Design review of the part built by this model. Coordinates are the model's own, in mm. Coordinates: 2 decimals unless noted, no trailing zeros. Loops run counter-clockwise (first coordinate to the right, second up) from the corner with the lowest first, then second, coordinate; pieces in that order, holes last.
Q1. Add section C-C on x = -8. Give the boundary of the cut face in (y, z) (3 decimals), and give its area (3 significant figures).
Q2. Add section D-D on y = 35.5. Give the boundary of the cut face in (x, z) (3 decimals), and give its area (3 significant figures).
Q3. For P1, Ø13, axis at x = 0, y = 0, coming from the +Z side; P2, Ø4, axis at x = -53.74, y = 48.92, coming from the +Z side; P3, Ø5, axis at x = -40, y = 0, coming from the +Z side; P4, Ø6, axis at x = 0, y = -8, coming from the +Z side (3 decimals), all flat-tipped, find the tip position at first contact; note any pin that passes through.
Q4. Add section B-B on y = 8. Give the boundary of the cut face in (x, z) (3 decimals), and give its area (3 significant figures).
Q5. Wall thickness on probe 1 along X at (y, z) = (47, -0.3); probe 2 along Y at (x, z) = (-68, -1.2); probe 3 along Y at (x, z) = (-57, -1.9): over which ranges is each line inside the solid? List them lowest first.
Q6. Draft analysis for pull direction Y (two halves, no side actions). For faces 1 (the face through (16, 7, -2)), 2 (the face through (-51, 54.5, -2)), 3 (the face through (-67.64, 48.99, -2.37)), state which applies: released by +Y, released by -Y, zero draft, split by the parting line, or undercut.
Q7. Add section A-A on x = -64. Give the boundary of the cut face in (y, z) (3 decimals), and give its area (3 significant figures).
```python
from build123d import *

# Parameters (mm, degrees)
SKETCH1_R                                       = 4
BOSS_EXTRUDE1_DEPTH                             = 3.175
CSK_FOR_M3_FLAT_HEAD_MACHINE_SCREW1_D           = 3.2
CSK_FOR_M3_FLAT_HEAD_MACHINE_SCREW1_CSINK_D     = 6.3
CSK_FOR_M3_FLAT_HEAD_MACHINE_SCREW1_CSINK_ANGLE = 90
F_31_64_0_48438_DIAMETER_HOLE1_D                = 12.303252
CSK_FOR_6_FLAT_HEAD_MACHINE_SCREW1_AT_2_COUNT   = 2
CSK_FOR_6_FLAT_HEAD_MACHINE_SCREW1_AT_2_PITCH   = 11.313708499
CSK_FOR_6_FLAT_HEAD_MACHINE_SCREW1_AT_3_COUNT   = 2
CSK_FOR_6_FLAT_HEAD_MACHINE_SCREW1_AT_3_PITCH   = 16
CSK_FOR_6_FLAT_HEAD_MACHINE_SCREW1_AT_4_COUNT   = 2
CSK_FOR_6_FLAT_HEAD_MACHINE_SCREW1_AT_4_PITCH   = 11.313708499
F_6_32_TAPPED_HOLE1_D                           = 2.7051
CSK_FOR_6_FLAT_HEAD_MACHINE_SCREW2_AT_2_COUNT   = 2
CSK_FOR_6_FLAT_HEAD_MACHINE_SCREW2_AT_2_PITCH   = 11.313708499
CSK_FOR_6_FLAT_HEAD_MACHINE_SCREW2_AT_3_COUNT   = 2
CSK_FOR_6_FLAT_HEAD_MACHINE_SCREW2_AT_3_PITCH   = 32
CSK_FOR_6_FLAT_HEAD_MACHINE_SCREW2_AT_4_COUNT   = 2
CSK_FOR_6_FLAT_HEAD_MACHINE_SCREW2_AT_4_PITCH   = 25.298221281
CSK_FOR_6_FLAT_HEAD_MACHINE_SCREW2_AT_5_COUNT   = 2
CSK_FOR_6_FLAT_HEAD_MACHINE_SCREW2_AT_5_PITCH   = 11.313708499


with BuildPart() as part:
    # Sketch1 → Boss-Extrude1 (new body)
    with BuildSketch(Plane.XY):
        Polygon((16, -16), (-80.487803669, -16), (-80.487803669, 46.5), (-72.487803669, 54.5), (-28.507138544, 54.5), (16, 28.803791581), align=None)
        Circle(SKETCH1_R, mode=Mode.SUBTRACT)
    extrude(amount=-BOSS_EXTRUDE1_DEPTH)

    # CSK for M3 Flat Head Machine Screw1 (through all)
    with Locations(Plane.XY):
        with Locations((-69.237803669, 48.923393759), (-53.737803669, 48.923393759), (-45.987803669, 35.5), (-53.737803669, 22.076606241), (-69.237803669, 22.076606241), (-76.987803669, 35.5)):
            CounterSinkHole(CSK_FOR_M3_FLAT_HEAD_MACHINE_SCREW1_D / 2, CSK_FOR_M3_FLAT_HEAD_MACHINE_SCREW1_CSINK_D / 2, counter_sink_angle=CSK_FOR_M3_FLAT_HEAD_MACHINE_SCREW1_CSINK_ANGLE)

    # 31_64 _0.48438_ Diameter Hole1 (through all)
    with Locations(Plane.XY):
        with Locations((-55.425625842, 32)):
            Hole(F_31_64_0_48438_DIAMETER_HOLE1_D / 2)

    # Sketch8 → CSK for _6 Flat Head Machine Screw1 (revolve, cut)
    with BuildSketch(Plane(origin=(0, 8, 0), x_dir=(0, -1, 0), z_dir=(1, 0, 0))):
        Polygon((0, 0), (0, 3.175), (1.8288, 3.175), (1.8288, 1.972306634), (3.5433, 0), align=None)
    csk_for_6_flat_head_machine_screw1 = revolve(axis=Axis((0, 8, 6.35), (0, 0, -1)), mode=Mode.SUBTRACT)

    # CSK for _6 Flat Head Machine Screw1 at 2: CSK for _6 Flat Head Machine Screw1 ×2
    with Locations(*[Vector(-0.707106781, -0.707106781, 0) * (i * CSK_FOR_6_FLAT_HEAD_MACHINE_SCREW1_AT_2_PITCH) for i in range(1, CSK_FOR_6_FLAT_HEAD_MACHINE_SCREW1_AT_2_COUNT)]):
        add(csk_for_6_flat_head_machine_screw1, mode=Mode.SUBTRACT)

    # CSK for _6 Flat Head Machine Screw1 at 3: CSK for _6 Flat Head Machine Screw1 ×2
    with Locations(*[(0, -i * CSK_FOR_6_FLAT_HEAD_MACHINE_SCREW1_AT_3_PITCH, 0) for i in range(1, CSK_FOR_6_FLAT_HEAD_MACHINE_SCREW1_AT_3_COUNT)]):
        add(csk_for_6_flat_head_machine_screw1, mode=Mode.SUBTRACT)

    # CSK for _6 Flat Head Machine Screw1 at 4: CSK for _6 Flat Head Machine Screw1 ×2
    with Locations(*[Vector(0.707106781, -0.707106781, 0) * (i * CSK_FOR_6_FLAT_HEAD_MACHINE_SCREW1_AT_4_PITCH) for i in range(1, CSK_FOR_6_FLAT_HEAD_MACHINE_SCREW1_AT_4_COUNT)]):
        add(csk_for_6_flat_head_machine_screw1, mode=Mode.SUBTRACT)

    # 6-32 Tapped Hole1 (through all)
    with Locations(Plane.XY):
        with Locations((-72, 0), (-32, -8), (-64, -8)):
            Hole(F_6_32_TAPPED_HOLE1_D / 2)

    # Sketch13 → CSK for _6 Flat Head Machine Screw2 (revolve, cut)
    with BuildSketch(Plane(origin=(-32, 8, 0), x_dir=(0, -1, 0), z_dir=(1, 0, 0))):
        Polygon((0, 0), (0, 3.175), (1.8288, 3.175), (1.8288, 1.972306634), (3.5433, 0), align=None)
    csk_for_6_flat_head_machine_screw2 = revolve(axis=Axis((-32, 8, 6.35), (0, 0, -1)), mode=Mode.SUBTRACT)

    # CSK for _6 Flat Head Machine Screw2 at 2: CSK for _6 Flat Head Machine Screw2 ×2
    with Locations(*[Vector(0.707106781, -0.707106781, 0) * (i * CSK_FOR_6_FLAT_HEAD_MACHINE_SCREW2_AT_2_PITCH) for i in range(1, CSK_FOR_6_FLAT_HEAD_MACHINE_SCREW2_AT_2_COUNT)]):
        add(csk_for_6_flat_head_machine_screw2, mode=Mode.SUBTRACT)

    # CSK for _6 Flat Head Machine Screw2 at 3: CSK for _6 Flat Head Machine Screw2 ×2
    with Locations(*[(-i * CSK_FOR_6_FLAT_HEAD_MACHINE_SCREW2_AT_3_PITCH, 0, 0) for i in range(1, CSK_FOR_6_FLAT_HEAD_MACHINE_SCREW2_AT_3_COUNT)]):
        add(csk_for_6_flat_head_machine_screw2, mode=Mode.SUBTRACT)

    # CSK for _6 Flat Head Machine Screw2 at 4: CSK for _6 Flat Head Machine Screw2 ×2
    with Locations(*[Vector(-0.948683298, -0.316227766, 0) * (i * CSK_FOR_6_FLAT_HEAD_MACHINE_SCREW2_AT_4_PITCH) for i in range(1, CSK_FOR_6_FLAT_HEAD_MACHINE_SCREW2_AT_4_COUNT)]):
        add(csk_for_6_flat_head_machine_screw2, mode=Mode.SUBTRACT)

    # CSK for _6 Flat Head Machine Screw2 at 5: CSK for _6 Flat Head Machine Screw2 ×2
    with Locations(*[Vector(-0.707106781, -0.707106781, 0) * (i * CSK_FOR_6_FLAT_HEAD_MACHINE_SCREW2_AT_5_PITCH) for i in range(1, CSK_FOR_6_FLAT_HEAD_MACHINE_SCREW2_AT_5_COUNT)]):
        add(csk_for_6_flat_head_machine_screw2, mode=Mode.SUBTRACT)


solid = part.part
```
Entries:
1. outline: (-16, -3.175) - (-1.829, -3.175) - (-1.829, -1.972) - (-3.543, 0) - (-16, 0) - close; (1.829, -3.175) - (42.66, -3.175) - (42.66, 0) - (3.543, 0) - (1.829, -1.972) - close
1. area: 171 mm2
2. outline: (-80.488, -3.175) - (-78.588, -3.175) - (-78.588, -1.55) - (-80.138, 0) - (-80.488, 0) - close; (-75.388, -3.175) - (-60.485, -3.175) - (-60.485, 0) - (-73.838, 0) - (-75.388, -1.55) - close; (-50.367, -3.175) - (-47.588, -3.175) - (-47.588, -1.55) - (-49.138, 0) - (-50.367, 0) - close; (-44.388, -3.175) - (4.402, -3.175) - (4.402, 0) - (-42.838, 0) - (-44.388, -1.55) - close
2. area: 212 mm2
3. P1: stops at z = 0
3. P2: stops at z = -1.15
3. P3: stops at z = -1.2
3. P4: stops at z = -0.625
4. outline: (-80.488, -3.175) - (-65.829, -3.175) - (-65.829, -1.972) - (-67.543, 0) - (-80.488, 0) - close; (-62.171, -3.175) - (-33.829, -3.175) - (-33.829, -1.972) - (-35.543, 0) - (-60.457, 0) - (-62.171, -1.972) - close; (-30.171, -3.175) - (-1.829, -3.175) - (-1.829, -1.972) - (-3.543, 0) - (-28.457, 0) - (-30.171, -1.972) - close; (1.829, -3.175) - (16, -3.175) - (16, 0) - (3.543, 0) - (1.829, -1.972) - close
4. area: 261 mm2
5. probe 1: x = -79.99 to -71.34, -67.13 to -55.84, -51.63 to -15.52
5. probe 2: y = -16 to 20.57, 23.58 to 47.42, 50.43 to 54.5
5. probe 3: y = -16 to -1.61, 1.61 to 26.05, 37.95 to 54.5
6. face 1: zero draft
6. face 2: released by +Y
6. face 3: undercut
7. outline: (-16, -3.175) - (-9.353, -3.175) - (-9.353, 0) - (-16, 0) - close; (-6.647, -3.175) - (6.171, -3.175) - (6.171, -1.972) - (4.457, 0) - (-6.647, 0) - close; (9.829, -3.175) - (54.5, -3.175) - (54.5, 0) - (11.543, 0) - (9.829, -1.972) - close
7. area: 200 mm2
